```python
from build123d import *

# Parameters (mm, degrees)
SKETCH1_W            = 106.68
SKETCH1_H            = 27.94
BOSS_EXTRUDE1_DEPTH  = 63.5
CUT_EXTRUDE2_DEPTH   = 96.52
SKETCH38_W           = 40.02
SKETCH38_H           = 63.5
BOSS_EXTRUDE25_DEPTH = 6.66
SKETCH40_W           = 6.35
SKETCH40_H           = 63.5
BOSS_EXTRUDE26_DEPTH = 18.74
SKETCH41_W           = 6.35
SKETCH41_H           = 63.5
BOSS_EXTRUDE27_DEPTH = 18.74
SKETCH43_W           = 27.32
SKETCH43_H           = 17.89
BOSS_EXTRUDE28_DEPTH = 18.74
CUT_EXTRUDE13_DEPTH  = 10.5
SKETCH46_W           = 27.32
SKETCH46_H           = 4.8
BOSS_EXTRUDE29_DEPTH = 4.8
BOSS_EXTRUDE30_DEPTH = 33.36
BOSS_EXTRUDE31_DEPTH = 35.11
BOSS_EXTRUDE32_DEPTH = 35.11
SKETCH52_W           = 40.02
SKETCH52_H           = 53
BOSS_EXTRUDE33_DEPTH = 6.35
SKETCH55_W           = 2.54
SKETCH55_H           = 4.8
BOSS_EXTRUDE37_DEPTH = 35.11
SKETCH56_W           = 2.54
SKETCH56_H           = 4.8
BOSS_EXTRUDE38_DEPTH = 35.11
BOSS_EXTRUDE35_DEPTH = 10.5
BOSS_EXTRUDE36_DEPTH = 10.5


with BuildPart() as part:
    # Sketch1 → Boss-Extrude1 (new body)
    with BuildSketch(Plane(origin=(0, 0, 0), x_dir=(1, 0, 0), z_dir=(0, 1, 0))):
        with Locations((53.34, -13.97)):
            Rectangle(SKETCH1_W, SKETCH1_H)
    extrude(amount=BOSS_EXTRUDE1_DEPTH)

    # Sketch2 → Cut-Extrude2 (cut)
    with BuildSketch(Plane.ZY):
        with BuildLine():
            Line((6.35, 50.8), (6.35, 6.35))
            Line((6.35, 6.35), (21.59, 6.35))
            Line((21.59, 6.35), (21.59, 50.8))
            add(Edge.make_bspline(
                [(6.35, 50.8), (13.97, 66.04), (21.59, 50.8)],
                knots=[0, 0, 0, 1, 1, 1], degree=2))
        make_face()
    extrude(amount=-CUT_EXTRUDE2_DEPTH, mode=Mode.SUBTRACT)

    # Sketch38 → Boss-Extrude25 (add)
    with BuildSketch(Plane(origin=(0, 0, 0), x_dir=(-1, 0, 0), z_dir=(0, 0, -1))):
        with Locations((-53.34, 31.75)):
            Rectangle(SKETCH38_W, SKETCH38_H)
    boss_extrude25 = extrude(amount=BOSS_EXTRUDE25_DEPTH)

    # Sketch40 → Boss-Extrude26 (add)
    with BuildSketch(Plane(origin=(0, 0, -6.66), x_dir=(-1, 0, 0), z_dir=(0, 0, -1))):
        with Locations((-70.175, 31.75)):
            Rectangle(SKETCH40_W, SKETCH40_H)
    boss_extrude26 = extrude(amount=BOSS_EXTRUDE26_DEPTH)

    # Sketch41 → Boss-Extrude27 (add)
    with BuildSketch(Plane(origin=(0, 0, -6.66), x_dir=(-1, 0, 0), z_dir=(0, 0, -1))):
        with Locations((-36.505, 31.75)):
            Rectangle(SKETCH41_W, SKETCH41_H)
    boss_extrude27 = extrude(amount=BOSS_EXTRUDE27_DEPTH)

    # Sketch43 → Boss-Extrude28 (add)
    with BuildSketch(Plane(origin=(0, 0, -6.66), x_dir=(-1, 0, 0), z_dir=(0, 0, -1))):
        with Locations((-53.34, 8.945)):
            Rectangle(SKETCH43_W, SKETCH43_H)
    boss_extrude28 = extrude(amount=BOSS_EXTRUDE28_DEPTH)

    # Sketch44 → Cut-Extrude13 (cut)
    with BuildSketch(Plane(origin=(0, 63.5, 0), x_dir=(1, 0, 0), z_dir=(0, 1, 0))):
        Polygon((73.35, 0), (33.33, 0), (33.33, 25.4), (39.68, 25.4), (39.68, 6.66), (67, 6.66), (67, 25.4), (73.35, 25.4), align=None)
    cut_extrude13 = extrude(amount=-CUT_EXTRUDE13_DEPTH, mode=Mode.SUBTRACT)

    # Sketch46 → Boss-Extrude29 (add)
    with BuildSketch(Plane(origin=(0, 0, -6.66), x_dir=(-1, 0, 0), z_dir=(0, 0, -1))):
        with Locations((-53.34, 50.6)):
            Rectangle(SKETCH46_W, SKETCH46_H)
    boss_extrude29 = extrude(amount=BOSS_EXTRUDE29_DEPTH)

    # Sketch48 → Boss-Extrude30 (add)
    with BuildSketch(Plane(origin=(39.68, 0, 0), x_dir=(0, 0, -1), z_dir=(1, 0, 0))):
        Polygon((11.46, 48.2), (6.66, 39.7), (6.66, 48.2), align=None)
    boss_extrude30 = extrude(amount=BOSS_EXTRUDE30_DEPTH)

    # Sketch50 → Boss-Extrude31 (add)
    with BuildSketch(Plane(origin=(0, 53, 0), x_dir=(1, 0, 0), z_dir=(0, 1, 0))):
        Polygon((64.46, 11.46), (67, 25.4), (67, 11.46), align=None)
    boss_extrude31 = extrude(amount=-BOSS_EXTRUDE31_DEPTH)

    # Sketch51 → Boss-Extrude32 (add)
    with BuildSketch(Plane(origin=(0, 53, 0), x_dir=(1, 0, 0), z_dir=(0, 1, 0))):
        Polygon((42.22, 11.46), (39.68, 11.46), (39.68, 25.4), align=None)
    boss_extrude32 = extrude(amount=-BOSS_EXTRUDE32_DEPTH)

    # Sketch52 → Boss-Extrude33 (add)
    with BuildSketch(Plane(origin=(0, 0, -25.4), x_dir=(-1, 0, 0), z_dir=(0, 0, -1))):
        with Locations((-53.34, 26.5)):
            Rectangle(SKETCH52_W, SKETCH52_H)
    boss_extrude33 = extrude(amount=BOSS_EXTRUDE33_DEPTH)

    # Sketch55 → Boss-Extrude37 (add)
    with BuildSketch(Plane(origin=(0, 17.89, 0), x_dir=(1, 0, 0), z_dir=(0, 1, 0))):
        with Locations((65.73, 9.06)):
            Rectangle(SKETCH55_W, SKETCH55_H)
    boss_extrude37 = extrude(amount=BOSS_EXTRUDE37_DEPTH)

    # Sketch56 → Boss-Extrude38 (add)
    with BuildSketch(Plane(origin=(0, 17.89, 0), x_dir=(1, 0, 0), z_dir=(0, 1, 0))):
        with Locations((40.95, 9.06)):
            Rectangle(SKETCH56_W, SKETCH56_H)
    boss_extrude38 = extrude(amount=BOSS_EXTRUDE38_DEPTH)

    # Mirror5: Boss-Extrude25, Boss-Extrude26, Boss-Extrude27, Boss-Extrude28, Cut-Extrude13, Boss-Extrude29, Boss-Extrude30, Boss-Extrude31, Boss-Extrude32, Boss-Extrude33, Boss-Extrude37, Boss-Extrude38 across plane
    add(boss_extrude25.mirror(Plane(origin=(0, 0, 13.97), x_dir=(1, 0, 0), z_dir=(0, 0, -1))))
    add(boss_extrude26.mirror(Plane(origin=(0, 0, 13.97), x_dir=(1, 0, 0), z_dir=(0, 0, -1))))
    add(boss_extrude27.mirror(Plane(origin=(0, 0, 13.97), x_dir=(1, 0, 0), z_dir=(0, 0, -1))))
    add(boss_extrude28.mirror(Plane(origin=(0, 0, 13.97), x_dir=(1, 0, 0), z_dir=(0, 0, -1))))
    add(cut_extrude13.mirror(Plane(origin=(0, 0, 13.97), x_dir=(1, 0, 0), z_dir=(0, 0, -1))), mode=Mode.SUBTRACT)
    add(boss_extrude29.mirror(Plane(origin=(0, 0, 13.97), x_dir=(1, 0, 0), z_dir=(0, 0, -1))))
    add(boss_extrude30.mirror(Plane(origin=(0, 0, 13.97), x_dir=(1, 0, 0), z_dir=(0, 0, -1))))
    add(boss_extrude31.mirror(Plane(origin=(0, 0, 13.97), x_dir=(1, 0, 0), z_dir=(0, 0, -1))))
    add(boss_extrude32.mirror(Plane(origin=(0, 0, 13.97), x_dir=(1, 0, 0), z_dir=(0, 0, -1))))
    add(boss_extrude33.mirror(Plane(origin=(0, 0, 13.97), x_dir=(1, 0, 0), z_dir=(0, 0, -1))))
    add(boss_extrude37.mirror(Plane(origin=(0, 0, 13.97), x_dir=(1, 0, 0), z_dir=(0, 0, -1))))
    add(boss_extrude38.mirror(Plane(origin=(0, 0, 13.97), x_dir=(1, 0, 0), z_dir=(0, 0, -1))))

    # Sketch53 → Boss-Extrude35 (add)
    with BuildSketch(Plane(origin=(0, 53, 0), x_dir=(1, 0, 0), z_dir=(0, 1, 0))):
        Polygon((64.46, 11.46), (39.68, 0), (73.35, 0), (73.35, 11.539525475), align=None)
    extrude(amount=BOSS_EXTRUDE35_DEPTH)

    # Sketch54 → Boss-Extrude36 (add)
    with BuildSketch(Plane(origin=(0, 53, 0), x_dir=(1, 0, 0), z_dir=(0, 1, 0))):
        Polygon((42.22, -39.4), (33.33, -39.4), (33.33, -27.94), (67, -27.94), align=None)
    extrude(amount=BOSS_EXTRUDE36_DEPTH)


solid = part.part
```
Geometry: final body of the model. Coordinates: model frame, mm. A direction names the side the tool comes from. Coordinates: 2 decimals unless noted, no trailing zeros. Order: outer loops, then holes, each group sorted by start corner. A loop starts at its lowest first (then second) coordinate and runs counter-clockwise, first axis right, second up. Notation, with made-up numbers: (-18.75, 87.25) -> (39.25, 87.25) arc R17 cw to (39.25, 97.25) -> close; hole circle Ø1 at (-25.5, -28). An arc over 180 degrees is marked (long way). Answer in a Markdown table with one row per item.
Item 1: Contact query for flat-ended pins moving along their axis: P1, Ø5.5, axis at y = 35, z = 36, coming from the -X side; P2, Ø6, axis at x = 11.5, z = 22, coming from the -Y side; P3, Ø8, axis at x = 17, y = 19, coming from the +Z side; P4, Ø8, axis at x = 64, z = 49.5, coming from the +Y side. Output: stop coordinate, or through.
Return value:
| item | result |
|---|---|
| P1 | stops at x = 33.33 |
| P2 | stops at y = 0 |
| P3 | stops at z = 27.94 |
| P4 | stops at y = 53 |
Item 2: Section B-B on z = 38. Output: boundary loops of the cut face in (x, y), plus the area to 3 significant figures.
Return value:
| item | result |
|---|---|
| outline | (33.33, 0) -> (73.35, 0) -> (73.35, 53) -> (45.25, 53) -> (45.25, 63.5) -> (33.33, 63.5) -> close; hole (42.22, 17.89) -> (64.46, 17.89) -> (64.46, 45.72) -> (42.22, 45.72) -> close |
| area | 1,630 mm² |
Item 3: Ray query, L1, parallel to Z at x = 50.5, y = 26; L2, parallel to Z at x = 12.5, y = 11.5; L3, parallel to Z at x = 49, y = 15. Return the intervals inside material, ascending.
Return value:
| item | result |
|---|---|
| L1 | z = -31.75 to -25.4, -6.66 to 6.35, 21.59 to 34.6, 53.34 to 59.69 |
| L2 | z = 0 to 6.35, 21.59 to 27.94 |
| L3 | z = -31.75 to 6.35, 21.59 to 59.69 |
Item 4: Access query for faces 1 (the flat face through (65.71, 35.69, -18.33)), 2 (the flat face through (53.184, 44.01, 37.034)), 3 (the flat face through (73.35, 31, -16)), 4 (the flat face through (33.33, 31, 44)). Directions: +Z, -Z, +X, -X, +Y, -Y. A direction counts if a zero-diameter tool reaches every point of the face in a straight line with its end or side. Return the directions, or none.
Return value:
| item | result |
|---|---|
| face 1 | +Y |
| face 2 | none |
| face 3 | -Z, +X, +Y, -Y |
| face 4 | +Z, -X, +Y, -Y |
Item 5: Section A-A on y = 24. Output: boundary loops of the cut face in (x, z).
Return value:
| item | result |
|---|---|
| outline | (0, 0) -> (33.33, 0) -> (33.33, -31.75) -> (73.35, -31.75) -> (73.35, 0) -> (106.68, 0) -> (106.68, 27.94) -> (73.35, 27.94) -> (73.35, 59.69) -> (33.33, 59.69) -> (33.33, 27.94) -> (0, 27.94) -> (0, 21.59) -> (96.52, 21.59) -> (96.52, 6.35) -> (0, 6.35) -> close; hole (39.68, -25.4) -> (67, -25.4) -> (64.46, -11.46) -> (64.46, -6.66) -> (42.22, -6.66) -> (42.22, -11.46) -> close; hole (39.68, 53.34) -> (42.22, 39.4) -> (42.22, 34.6) -> (64.46, 34.6) -> (64.46, 39.4) -> (67, 53.34) -> close |
Item 6: Section C-C on y = 13.5. Output: boundary loops of the cut face in (x, z).
Return value:
| item | result |
|---|---|
| outline | (0, 0) -> (33.33, 0) -> (33.33, -31.75) -> (73.35, -31.75) -> (73.35, 0) -> (106.68, 0) -> (106.68, 27.94) -> (73.35, 27.94) -> (73.35, 59.69) -> (33.33, 59.69) -> (33.33, 27.94) -> (0, 27.94) -> (0, 21.59) -> (96.52, 21.59) -> (96.52, 6.35) -> (0, 6.35) -> close |
Item 7: Draft query along Z for faces 5 (the flat face through (90, 31, 0)), 6 (the flat face through (65.71, 35.69, 46.27)), 7 (the flat face through (54, 63.5, 14)). Return one class per face: released by +Z, released by -Z, zero draft, split by the parting line, or undercut.
Return value:
| item | result |
|---|---|
| face 5 | released by -Z |
| face 6 | undercut |
| face 7 | zero draft |
